The listing builds one solid part. Answer for the finished solid, in the listing's coordinates (mm). A direction names the side the tool comes from. Round coordinates to 2 decimals unless told otherwise and drop trailing zeros. Loops run counter-clockwise (first coordinate to the right, second up) from the corner with the lowest first, then second, coordinate; pieces in that order, holes last. Notation, with made-up numbers: M 37.5,43.25 L 69.5,43.25 A27 ccw 69.5,76.25 Z; hole C 32.25,-5.75 d9. An arc over 180 degrees is marked long. Put each result on its own line as item: value. Start each with the question number.
(1) Which of the six approach directions +Z, -Z, +X, -X, +Y, -Y give full straight-line access (tool end or side, diameter ignored) to faces 1 (the face through (-5.563, 3.062, 14.275)), 2 (the face through (-2.184, -1.237, 14.275))?
(2) Section C-C, the plane x = 5.25 is taken. Determine the outline of the cut face in (y, z).
(3) Straight lines are drawn through the part: line 1 (X direction, y = -2, z = 21.75); line 2 (X direction, y = 1.5, z = 8.75); line 3 (Y direction, x = 0.5, z = 27.75). For each, find the intervals that lie inside material, in ascending order.
(4) Section A-A, the plane z = 4 is taken. Determine the outline of the cut face in (x, y), then the cut area to 3 significant figures.
(5) Section D-D, the plane y = -3.5 is taken. Determine the outline of the cut face in (x, z).
(6) Section B-B, the plane y = 0.5 is taken. Determine the outline of the cut face in (x, z).
(7) Flat-ended cylindrical pins translate along their axes: P1, Ø2.5, axis at x = 0.5, z = 17, coming from the -Y side; P2, Ø5, axis at y = 3.5, z = 16, coming from the -X side; P3, Ø2, axis at x = 5.5, z = 19.5, coming from the +Y side. Find the tip coordinate at first contact, or state that the pin passes through.
(8) Determine the mould class of faces 3 (the face through (0, -3, 0)), 4 (the face through (0, -2.51, 14)), 5 (the face through (2.164, -1.273, 14.275)), 6 (the face through (5.43, 3.29, 14.28)) for opening direction X: released by +X, released by -X, zero draft, split by the parting line, or undercut.
```python
from build123d import *

# Parameters (mm, degrees)
BOSS_EXTRUDE2_DEPTH = 28.956


with BuildPart() as part:
    # Sketch4 → Boss-Extrude2 (new body)
    # profile 1 of 2: a face of its own
    with BuildSketch(Plane.XY):
        Polygon((-3.483559495, -6.4519878), (3.845805592, -6.242844919), (7.329365088, 0.209142882), (3.483559495, 6.4519878), (-3.845805592, 6.242844919), (-7.329365088, -0.209142882), align=None)
        Polygon((2.306514325, -3.995), (4.613028651, 0), (2.306514325, 3.995), (-2.306514325, 3.995), (-4.613028651, 0), (-2.306514325, -3.995), align=None, mode=Mode.SUBTRACT)
    # profile 2 of 2: a face of its own
    with BuildSketch(Plane.XY):
        Polygon((-2.306514325, -3.995), (2.306514325, -3.995), (4.613028651, 0), (2.306514325, 3.995), (-2.306514325, 3.995), (-4.613028651, 0), align=None)
        Polygon((1.449149176, -2.51), (2.898298351, 0), (1.449149176, 2.51), (-1.449149176, 2.51), (-2.898298351, 0), (-1.449149176, -2.51), align=None, mode=Mode.SUBTRACT)
    extrude(amount=BOSS_EXTRUDE2_DEPTH)


solid = part.part
```
Recorded:
1. face 1: +Z, -Z, -X, +Y
1. face 2: +Z, -Z
2. outline: M -3.64,0 L 3.58,0 L 3.58,28.96 L -3.64,28.96 Z
3. line 1: x = -6.23 to -1.74, 1.74 to 6.14
3. line 2: x = -6.41 to -2.03, 2.03 to 6.53
3. line 3: y = -6.34 to -2.51, 2.51 to 6.37
4. outline: M -7.33,-0.21 L -3.48,-6.45 L 3.85,-6.24 L 7.33,0.21 L 3.48,6.45 L -3.85,6.24 Z; hole M -2.9,0 L -1.45,-2.51 L 1.45,-2.51 L 2.9,0 L 1.45,2.51 L -1.45,2.51 Z
4. area: 118 mm²
5. outline: M -5.3,0 L 5.33,0 L 5.33,28.96 L -5.3,28.96 Z
6. outline: M -6.95,0 L -2.61,0 L -2.61,28.96 L -6.95,28.96 Z; M 2.61,0 L 7.15,0 L 7.15,28.96 L 2.61,28.96 Z
7. P1: stops at y = -6.37
7. P2: stops at x = -6.68
7. P3: stops at y = 4.8
8. face 3: zero draft
8. face 4: undercut
8. face 5: undercut
8. face 6: released by +X
